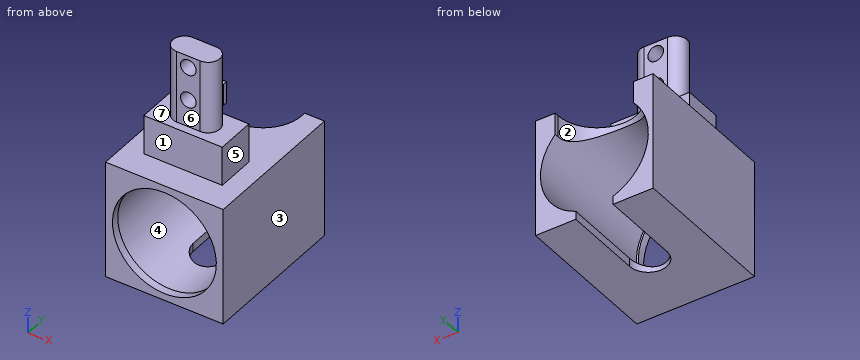
from build123d import *

# Parameters (mm, degrees)
SKETCH1_W               = 30
SKETCH1_H               = 36
BOSS_EXTRUDE1_DEPTH     = 30
SKETCH2_W               = 20
SKETCH2_H               = 10
BOSS_EXTRUDE2_DEPTH     = 10
BOSS_EXTRUDE3_DEPTH     = 18.5
CUT_EXTRUDE2_REACH      = 72.308
SKETCH4_R               = 13.75
CUT_EXTRUDE5_REACH      = 65.018
CUT_EXTRUDE5_END_RADIUS = 13.75
CUT_EXTRUDE6_REACH      = 40.066
CUT_EXTRUDE6_END_RADIUS = 13.75
CUT_EXTRUDE7_REACH      = 72.308
SKETCH9_R               = 2
SKETCH10_W              = 30
SKETCH10_H              = 30
BOSS_EXTRUDE4_DEPTH     = 2
CUT_EXTRUDE8_REACH      = 72.308
SKETCH11_R              = 13.25


with BuildPart() as part:
    # Sketch1 → Boss-Extrude1 (new body)
    with BuildSketch(Plane.XY):
        Rectangle(SKETCH1_W, SKETCH1_H)
    extrude(amount=BOSS_EXTRUDE1_DEPTH)

    # Sketch2 → Boss-Extrude2 (add)
    with BuildSketch(Plane.XY.offset(30)):
        with Locations((0, -8)):
            Rectangle(SKETCH2_W, SKETCH2_H)
    extrude(amount=BOSS_EXTRUDE2_DEPTH)

    # Sketch3 → Boss-Extrude3 (add)
    with BuildSketch(Plane.XY.offset(40)):
        with BuildLine():
            Line((-3, -5), (3, -5))
            ThreePointArc((3, -5), (6, -8), (3, -11))
            Line((3, -11), (-3, -11))
            ThreePointArc((-3, -11), (-6, -8), (-3, -5))
        make_face()
    extrude(amount=BOSS_EXTRUDE3_DEPTH)

    # Sketch4 → Cut-Extrude2 (cut, up to next)
    with BuildSketch(Plane(origin=(0, 18, 0), x_dir=(1, 0, 0), z_dir=(0, 1, 0)), mode=Mode.PRIVATE) as cut_extrude2_sk1:
        with Locations(Location((0, -15, 0), (0, 0, 270))):
            Circle(SKETCH4_R)
    cut_extrude2_tool1 = extrude(cut_extrude2_sk1.sketch, amount=-CUT_EXTRUDE2_REACH, mode=Mode.PRIVATE) & part.part
    add(cut_extrude2_tool1.solids().sort_by_distance((0, 18, 15))[0], mode=Mode.SUBTRACT)

    # Cut-Extrude5: up to this cylinder (the profile starts outside it)
    cut_extrude5_end = Plane(origin=(0, 7.875, 15), z_dir=(0, 1, 0)) * Cylinder(CUT_EXTRUDE5_END_RADIUS, 158.536, mode=Mode.PRIVATE)
    # Sketch6 → Cut-Extrude5 (cut, up to the surface)
    with BuildSketch(Plane(origin=(0, 0, 0), x_dir=(-1, 0, 0), z_dir=(0, 0, -1)), mode=Mode.PRIVATE) as cut_extrude5_sk1:
        with BuildLine():
            Line((-4.75, -2.25), (-4.75, 18))
            ThreePointArc((-4.75, 18), (0, 22.75), (4.75, 18))
            Line((4.75, 18), (4.75, -2.25))
            ThreePointArc((4.75, -2.25), (0, -7), (-4.75, -2.25))
        make_face()
    cut_extrude5_tool1 = extrude(cut_extrude5_sk1.sketch, amount=-CUT_EXTRUDE5_REACH, mode=Mode.PRIVATE) - cut_extrude5_end
    add(cut_extrude5_tool1.solids().sort_by_distance((0, 7.875, 0))[0], mode=Mode.SUBTRACT)

    # Cut-Extrude6: up to this cylinder (the profile starts outside it)
    cut_extrude6_end = Plane(origin=(0, 17.5, 15), z_dir=(0, 1, 0)) * Cylinder(CUT_EXTRUDE6_END_RADIUS, 108.632, mode=Mode.PRIVATE)
    # Sketch8 → Cut-Extrude6 (cut, up to the surface)
    with BuildSketch(Plane.XY.offset(30), mode=Mode.PRIVATE) as cut_extrude6_sk1:
        with BuildLine():
            Line((-10, 17), (-10, 18))
            ThreePointArc((-10, 18), (0, 28), (10, 18))
            Line((10, 18), (10, 17))
            ThreePointArc((10, 17), (0, 7), (-10, 17))
        make_face()
    cut_extrude6_tool1 = extrude(cut_extrude6_sk1.sketch, amount=-CUT_EXTRUDE6_REACH, mode=Mode.PRIVATE) - cut_extrude6_end
    add(cut_extrude6_tool1.solids().sort_by_distance((0, 17.5, 30))[0], mode=Mode.SUBTRACT)

    # Sketch9 → Cut-Extrude7 (cut, up to next)
    with BuildSketch(Plane.XZ.offset(18), mode=Mode.PRIVATE) as cut_extrude7_sk1:
        with Locations(Location((0, 55.5, 0), (0, 0, 270))):
            Circle(SKETCH9_R)
    cut_extrude7_tool1 = extrude(cut_extrude7_sk1.sketch, amount=-CUT_EXTRUDE7_REACH, mode=Mode.PRIVATE) & part.part
    # Sketch9 → Cut-Extrude7 (cut, up to next)
    with BuildSketch(Plane.XZ.offset(18), mode=Mode.PRIVATE) as cut_extrude7_sk2:
        with Locations(Location((0, 47, 0), (0, 0, 270))):
            Circle(SKETCH9_R)
    cut_extrude7_tool2 = extrude(cut_extrude7_sk2.sketch, amount=-CUT_EXTRUDE7_REACH, mode=Mode.PRIVATE) & part.part
    add(cut_extrude7_tool1.solids().sort_by_distance((0, -18, 55.5))[0], mode=Mode.SUBTRACT)
    add(cut_extrude7_tool2.solids().sort_by_distance((0, -18, 47))[0], mode=Mode.SUBTRACT)

    # Sketch10 → Boss-Extrude4 (add)
    with BuildSketch(Plane(origin=(0, -18, 0), x_dir=(-1, 0, 0), z_dir=(0, -1, 0))):
        with Locations((0, -15)):
            Rectangle(SKETCH10_W, SKETCH10_H)
    extrude(amount=BOSS_EXTRUDE4_DEPTH)

    # Sketch11 → Cut-Extrude8 (cut, up to next)
    with BuildSketch(Plane(origin=(0, -18, 0), x_dir=(1, 0, 0), z_dir=(0, 1, 0)), mode=Mode.PRIVATE) as cut_extrude8_sk1:
        with Locations(Location((0, -15, 0), (0, 0, 270))):
            Circle(SKETCH11_R)
    cut_extrude8_tool1 = extrude(cut_extrude8_sk1.sketch, amount=-CUT_EXTRUDE8_REACH, mode=Mode.PRIVATE) & part.part
    add(cut_extrude8_tool1.solids().sort_by_distance((0, -18, 15))[0], mode=Mode.SUBTRACT)


solid = part.part
Design review of the part built by this model. Coordinates are the model's own, in mm. Face numbers are marked on the shaded views. A direction names the side the tool comes from. Give positions to 0.01 mm unless a question says otherwise; leave off trailing zeros. Order: outer loops, then holes, each group sorted by start corner. A loop starts at its lowest first (then second) coordinate and runs counter-clockwise, first axis right, second up.
1. For pin 1 Ø2 at (x, z) = (5.5, 35) entering from +Y; pin 2 Ø1.8 at (x, z) = (1, 48.5) entering from -Y; pin 3 Ø6.5 at (x, z) = (0.5, 47.5) entering from +Y, all flat-tipped, find the tip position at first contact; note any pin that passes through.
Solution:
pin 1: stops at y = -3
pin 2: stops at y = -11
pin 3: stops at y = -5
2. Mouldability with a two-part tool opening along X and no side actions: class the marked faces 1, 2, 3 and 4 as +X half, -X half, draft (parallel to the pull), parting line (faces both ways), or undercut.
Solution:
face 1: draft
face 2: undercut
face 3: +X half
face 4: undercut
3. Add section C-C, the plane y = 5.5. State the section outline as (x, z) points, then the cut area to 3 significant figures.
Solution:
outline: (-15, 0) - (-4.75, 0) - (-4.75, 2.1) arc R13.75 cw (long way) to (4.75, 2.1) - (4.75, 0) - (15, 0) - (15, 30) - (-15, 30) - close
area: 292 mm2
4. Add section B-B, the plane x = -11.75. State the section outline as (y, z) points, then the cut area to 3 significant figures.
Solution:
outline: (-20, 0) - (18, 0) - (18, 7.86) - (-18, 7.86) - (-18, 8.88) - (-20, 8.88) - close; (-20, 21.12) - (-18, 21.12) - (-18, 22.14) - (18, 22.14) - (18, 30) - (-20, 30) - close
area: 601 mm2
5. Tool access review of the marked faces 5, 6 and 7: name each direction out of +Z, -Z, +X, -X, +Y, -Y from which nothing blocks a thin tool from reaching the whole face with its end or side.
Solution:
face 5: +Z, +X, +Y, -Y
face 6: +Z, +X, -X, -Y
face 7: +Z
6. Add section D-D, the plane z = 15. State the section outline as (x, y) points, then the cut area to 3 significant figures.
Solution:
outline: (-15, -20) - (-13.25, -20) - (-13.25, -18) - (-13.75, -18) - (-13.75, 18) - (-15, 18) - close; (13.25, -20) - (15, -20) - (15, 18) - (13.75, 18) - (13.75, -18) - (13.25, -18) - close
area: 97.0 mm2
7. Add section A-A, the plane z = 55.5. State the section outline as (x, y) points, then the cut area to 3 significant figures.
Solution:
outline: (-3, -11) - (-2, -11) - (-2, -5) - (-3, -5) arc R3 ccw to start; (2, -11) - (3, -11) arc R3 ccw to (3, -5) - (2, -5) - close
area: 40.3 mm2
8. To check wall thickness, follow L1, parallel to Z at x = -1.5, y = -10; L2, parallel to X at y = 1, z = 15; L3, parallel to Y at x = 0.5, z = 44. State the ranges of each line that lie inside material, in increasing order.
Solution:
L1: z = 0 to 1.33, 28.67 to 45.68, 48.32 to 54.18, 56.82 to 58.5
L2: x = -15 to -13.75, 13.75 to 15
L3: y = -11 to -5
